The model under review builds one solid part; all positions refer to its coordinate system, in mm. Face numbers are marked on the shaded views. Give positions to 0.01 mm unless a question says otherwise; leave off trailing zeros. Order: outer loops, then holes, each group sorted by start corner. A loop starts at its lowest first (then second) coordinate and runs counter-clockwise, first axis right, second up.
Autodesk Inventor part; units mm, degrees
ref_plane "Work Plane1" through (-49.5, -19.63, -109) normal (0, 0, -1) x (0, 1, 0)
ref_plane "Work Plane2" through (-47.0185, 3.2145, -3.5) normal (1, 0, 0) x (0, 1, 0)
ref_plane "YZ Plane" through (0, 0, 0) normal (1, 0, 0) x (0, 1, 0)
sketch "Sketch1" plane through (0, 0, 0) normal (0, 0, 1) x (1, 0, 0)
  line L0 (47.5, 19.63) -> (-47.5, 19.63)
  arc A0 (-47.5, 19.63) -> (-49.5, 17.63) centre (-47.5, 17.63) ccw
  line L1 (-49.5, 17.63) -> (-49.5, -19.63)
  line L2 (49.5, -19.63) -> (49.5, 17.63)
  arc A1 (49.5, 17.63) -> (47.5, 19.63) centre (47.5, 17.63) ccw
  line L3 (-49.5, -19.63) -> (-52, -19.63)
  line L4 (-52, -19.63) -> (-52, 20.13)
  line L5 (-50, 22.13) -> (50, 22.13)
  line L6 (52, 20.13) -> (52, -19.63)
  line L7 (52, -19.63) -> (49.5, -19.63)
  arc A2 (-50, 22.13) -> (-52, 20.13) centre (-50, 20.13) ccw
  arc A3 (52, 20.13) -> (50, 22.13) centre (50, 20.13) ccw
  dimension "d0" = 2.5
  dimension "d1" = 2.5
  dimension "d2" = 2.5
  dimension "d3" = 2
ref_plane "Work Plane1" through (-49.5, -19.63, -109) normal (0, 0, -1) x (0, 1, 0)
extrude "Extrusion1" add sketch "Sketch1" against normal up to surface (109 mm away)
sketch "Sketch2" plane through (-50, 22.13, 0) normal (0, 1, 0) x (1, 0, 0)
  circle A0 centre (39.65, 50.5) radius 18.5 construction
  line L0 (58.85, 79.4) -> (20.45, 79.4) construction
  line L1 (20.45, 79.4) -> (20.45, 21.6) construction
  line L2 (58.85, 21.6) -> (58.85, 79.4) construction
  line L3 (20.45, 21.6) -> (58.85, 21.6) construction
  line L4 (20.15, 23.6) -> (20.15, 77.4) construction
  line L5 (59.15, 77.4) -> (59.15, 23.6) construction
  line L6 (20.15, 21.6) -> (59.15, 21.6) construction
  line L7 (59.15, 79.4) -> (20.15, 79.4) construction
  line L8 (20.15, 21.6) -> (59.15, 21.6)
  line L9 (59.15, 21.6) -> (59.15, 79.4)
  line L10 (59.15, 79.4) -> (20.15, 79.4)
  line L11 (20.15, 79.4) -> (20.15, 21.6)
  line L12 (59.65, 79.4) -> (19.65, 79.4)
  line L13 (19.65, 79.4) -> (19.65, 21.6)
  line L14 (19.65, 21.6) -> (59.65, 21.6)
  line L15 (59.65, 21.6) -> (59.65, 79.4)
  point P0 (50, 0)
  point P1 (59.65, 50.5)
  point P2 (59.15, 79.4)
  dimension "d43" = 40
  dimension "d44" = 39
  dimension "d45" = 0.5
extrude "Extrusion2" cut sketch "Sketch2" against normal up to surface (2.5 mm away)
chamfer "Chamfer1" distance 2.5 angle 45 4 edges at (-10.35, 22.13, -79.4) (-30.35, 22.13, -50.5) (9.65, 22.13, -50.5) (-10.35, 22.13, -21.6)
sketch "Sketch3" plane through (-52, -19.63, 0) normal (-1, 0, 0) x (0, 0, 1)
  line L0 (-94, 9.5) -> (-94, 37.26)
  arc A0 (-92, 39.26) -> (-94, 37.26) centre (-92, 37.26) ccw
  line L1 (-92, 39.26) -> (-17, 39.26)
  arc A1 (-15, 37.26) -> (-17, 39.26) centre (-17, 37.26) ccw
  line L2 (-15, 37.26) -> (-15, 9.5)
  line L3 (-94, 9.5) -> (-94, 0)
  line L4 (0, 0) -> (-109, 0) construction
  line L5 (-15, 9.5) -> (-15, 0)
  line L6 (-94, 0) -> (-15, 0)
  circle A2 centre (-98, 6.25) radius 1.5 construction
  circle A3 centre (-11, 6.25) radius 1.5 construction
  circle A4 centre (-98, 6.25) radius 1.75
  circle A5 centre (-11, 6.25) radius 1.75
  point P0 (0, 19.63)
  dimension "d13" = 3.5
  dimension "d14" = 3.5
ref_plane "Work Plane2" through (-47.0185, 3.2145, -3.5) normal (1, 0, 0) x (0, 1, 0)
extrude "Extrusion3" cut sketch "Sketch3" against normal up to surface (4.9815 mm away)
sketch "Sketch4" plane through (52, -19.63, 0) normal (1, 0, 0) x (0, 0, -1)
  circle A0 centre (98, 6.25) radius 1.5 construction
  circle A1 centre (11, 6.25) radius 1.5 construction
  arc A2 (72.9, 14.47) -> (72.9168, 14.38) centre (73.1508, 14.4702) ccw construction
  line L0 (72.9, 16.76) -> (72.9, 14.47) construction
  line L1 (72.9, 16.76) -> (72.9, 18.76) construction
  line L2 (72.9, 22.14) -> (72.9, 18.76) construction
  arc A3 (73.15, 22.39) -> (72.9, 22.14) centre (73.15, 22.14) ccw construction
  line L3 (73.15, 22.39) -> (85.55, 22.39) construction
  arc A4 (85.8, 22.14) -> (85.55, 22.39) centre (85.55, 22.14) ccw construction
  line L4 (85.8, 22.14) -> (85.8, 18.76) construction
  line L5 (85.8, 18.76) -> (85.8, 16.76) construction
  line L6 (85.8, 16.76) -> (85.8, 14.47) construction
  arc A5 (85.7832, 14.38) -> (85.8, 14.47) centre (85.5492, 14.4702) ccw construction
  line L7 (85.7832, 14.38) -> (86.5, 14.38) construction
  line L8 (86.5, 14.38) -> (86.5, 12.03) construction
  line L9 (81.88, 12.03) -> (86.5, 12.03) construction
  line L10 (81.88, 12.03) -> (81.88, 11.42) construction
  line L11 (81.88, 11.42) -> (86.45, 11.42) construction
  line L12 (87.2, 11.42) -> (86.45, 11.42) construction
  line L13 (87.2, 24.47) -> (87.2, 11.42) construction
  line L14 (87.2, 24.52) -> (87.2, 24.47) construction
  line L15 (87.2, 24.52) -> (71.7, 24.52) construction
  line L16 (71.7, 24.52) -> (71.7, 24.47) construction
  line L17 (71.7, 24.47) -> (71.7, 11.42) construction
  line L18 (71.7, 11.42) -> (72.45, 11.42) construction
  line L19 (72.45, 11.42) -> (76.82, 11.42) construction
  line L20 (76.82, 12.03) -> (76.82, 11.42) construction
  line L21 (72.3, 12.03) -> (76.82, 12.03) construction
  line L22 (72.3, 14.38) -> (72.3, 12.03) construction
  line L23 (72.3, 14.38) -> (72.9168, 14.38) construction
  line L24 (68.675, 20.9412) -> (68.975, 20.9412) construction
  line L25 (68.975, 20.9412) -> (68.975, 26.4362) construction
  arc A6 (68.975, 26.4362) -> (68.375, 27.0362) centre (68.375, 26.4362) ccw construction
  line L26 (68.375, 27.0362) -> (55.825, 27.0362) construction
  arc A7 (55.825, 27.0362) -> (55.225, 26.4362) centre (55.825, 26.4362) ccw construction
  line L27 (55.225, 26.4362) -> (55.225, 20.9412) construction
  line L28 (55.225, 20.9412) -> (55.525, 20.9412) construction
  line L29 (55.525, 26.4362) -> (55.525, 20.9412) construction
  arc A8 (55.825, 26.7362) -> (55.525, 26.4362) centre (55.825, 26.4362) ccw construction
  line L30 (68.375, 26.7362) -> (55.825, 26.7362) construction
  arc A9 (68.675, 26.4362) -> (68.375, 26.7362) centre (68.375, 26.4362) ccw construction
  line L31 (68.675, 26.4362) -> (68.675, 20.9412) construction
  line L32 (51.675, 20.9412) -> (51.975, 20.9412) construction
  line L33 (51.975, 20.9412) -> (51.975, 26.4362) construction
  arc A10 (51.975, 26.4362) -> (51.375, 27.0362) centre (51.375, 26.4362) ccw construction
  line L34 (51.375, 27.0362) -> (38.825, 27.0362) construction
  arc A11 (38.825, 27.0362) -> (38.225, 26.4362) centre (38.825, 26.4362) ccw construction
  line L35 (38.225, 26.4362) -> (38.225, 20.9412) construction
  line L36 (38.225, 20.9412) -> (38.525, 20.9412) construction
  line L37 (38.525, 26.4362) -> (38.525, 20.9412) construction
  arc A12 (38.825, 26.7362) -> (38.525, 26.4362) centre (38.825, 26.4362) ccw construction
  line L38 (51.375, 26.7362) -> (38.825, 26.7362) construction
  arc A13 (51.675, 26.4362) -> (51.375, 26.7362) centre (51.375, 26.4362) ccw construction
  line L39 (51.675, 26.4362) -> (51.675, 20.9412) construction
  line L40 (3.1, 11.07) -> (101.9, 11.07) construction
  circle A14 centre (8.5, 17.57) radius 4
  circle A15 centre (11, 6.25) radius 1.75
  circle A16 centre (98, 6.25) radius 1.75
  line L41 (37.975, 27.2862) -> (52.225, 27.2862)
  line L42 (52.225, 27.2862) -> (52.225, 10.82)
  line L43 (52.225, 10.82) -> (37.975, 10.82)
  line L44 (37.975, 10.82) -> (37.975, 27.2862)
  line L45 (54.975, 27.2862) -> (69.225, 27.2862)
  line L46 (69.225, 27.2862) -> (69.225, 10.82)
  line L47 (69.225, 10.82) -> (54.975, 10.82)
  line L48 (54.975, 10.82) -> (54.975, 27.2862)
  line L49 (71.45, 24.72) -> (87.45, 24.72)
  line L50 (87.45, 24.72) -> (87.45, 10.82)
  line L51 (87.45, 10.82) -> (71.45, 10.82)
  line L52 (71.45, 10.82) -> (71.45, 24.72)
  line L53 (90.5, 13.2962) -> (90.5, 12.7462) construction
  line L54 (91.35, 13.7962) -> (91, 13.7962) construction
  line L55 (98, 13.7962) -> (97.6, 13.7962) construction
  line L56 (98.5, 13.2962) -> (98.5, 12.7462) construction
  line L57 (89.75, 14.2962) -> (99.25, 14.2962)
  line L58 (99.25, 14.2962) -> (99.25, 10.57)
  line L59 (99.25, 10.57) -> (89.75, 10.57)
  line L60 (89.75, 10.57) -> (89.75, 14.2962)
  line L61 (71.7, 24.47) -> (87.2, 24.47) construction
  line L62 (87.2, 24.47) -> (87.2, 11.07) construction
  line L63 (87.2, 11.07) -> (71.7, 11.07) construction
  line L64 (71.7, 11.07) -> (71.7, 24.47) construction
  circle A17 centre (8.5, 17.57) radius 3.2
  line L65 (19.46, 17.8062) -> (32.46, 17.8062) construction
  line L66 (16.81, 16.0562) -> (16.81, 16.7062) construction
  line L67 (33.71, 16.5312) -> (33.71, 12.5212) construction
  line L68 (18.4564, 11.8926) -> (16.9564, 13.3926) construction
  line L69 (16.56, 17.8062) -> (33.96, 17.8062)
  line L70 (33.96, 17.8062) -> (33.96, 10.82)
  line L71 (33.96, 10.82) -> (19.1755, 10.82)
  line L72 (19.1755, 10.82) -> (16.56, 13.4355)
  line L73 (16.56, 13.4355) -> (16.56, 17.8062)
  point P0 (0, 19.63)
  point P1 (17.8, 27.1262)
  point P2 (68.975, 23.6887)
  point P3 (91.175, 13.7962)
  point P4 (90.5, 13.0212)
  point P5 (98.5, 13.0212)
  point P6 (16.81, 16.3812)
  dimension "d15" = 8
  dimension "d16" = 3.5
  dimension "d17" = 3.5
  dimension "d23" = 0.25
  dimension "d24" = 0.25
  dimension "d25" = 0.25
  dimension "d26" = 0.25
  dimension "d27" = 0.25
  dimension "d28" = 0.25
  dimension "d29" = 0.25
  dimension "d30" = 0.25
  dimension "d31" = 0.25
  dimension "d32" = 0.25
  dimension "d33" = 0.25
  dimension "d34" = 0.5
  dimension "d35" = 0.5
  dimension "d36" = 0.75
  dimension "d37" = 0.75
  dimension "d46" = 0.25
  dimension "d47" = 0.25
  dimension "d49" = 0.25
  dimension "d50" = 0.25
  dimension "d51" = 0.25
  dimension "d52" = 0
extrude "Extrusion4" cut sketch "Sketch4" against normal up to surface (2.5 mm away) contours A14 | A15 | A16 | L41 L42 L43 L44 | L45 L46 L47 L48 | L49 L50 L51 L52 | L57 L58 L59 L60 | A17 | L69 L70 L71 L72 L73
chamfer "Chamfer2" distance 2 angle 45 4 edges at (52, -13.38, -9.25) (52, -13.38, -96.25) (-52, -13.38, -99.75) (-52, -13.38, -12.75)
equation "\"d1\" = d0"
equation "\"d2\" = d0"
equation "\"d45\" = -0.5 * d44 + 0.5 * d43"
equation "\"d14\" = d13"
equation "\"d17\" = d16"
equation "\"d23\" = d20"
equation "\"d24\" = d23"
equation "\"d25\" = d24"
equation "\"d26\" = d24"
equation "\"d28\" = d26"
equation "\"d29\" = d25"
equation "\"d30\" = d29"
equation "\"d31\" = d27"
equation "\"d32\" = d31"
equation "\"d33\" = d31"
equation "\"d34\" = d35"
equation "\"d20\" = d18"
properties part number "Shroud Top"
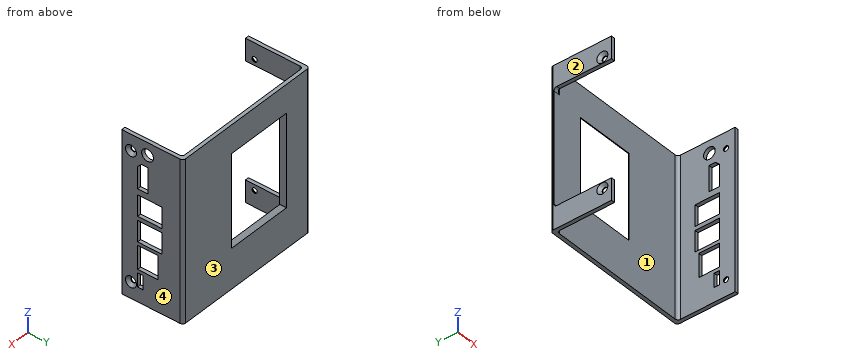
Item 1: Clearance check with flat-ended pins moving along their axes: pin 1 Ø1 at (x, z) = (28.5, -11.5) entering from -Y; pin 2 Ø5 at (y, z) = (-8.5, -75.5) entering from -X; pin 3 Ø0.8 at (x, z) = (50.5, -93) entering from +Y. State where each tip first meets the part, or that it passes through.
Values found:
pin 1: stops at y = 19.63
pin 2: stops at x = 49.5
pin 3: stops at y = 22.13
Item 2: Take a section at A-A (y = 15.5). Give the boundary of the cut face in (x, z).
Values found:
outline: (-52, -109) - (-49.5, -109) - (-49.5, -94) - (-52, -94) - close; (-52, -15) - (-49.5, -15) - (-49.5, 0) - (-52, 0) - close; (49.5, -109) - (52, -109) - (52, 0) - (49.5, 0) - close
Item 3: Take a section at B-B (z = -47). Give the number of separate pieces and of enclosed holes in the cut face, and give its area (3 significant figures).
Values found:
separate pieces: 3
enclosed holes: 0
area: 210 mm2
Item 4: Take a section at D-D (z = -11). Give the boundary of the cut face in (x, y).
Values found:
outline: (-52, -19.63) - (-49.5, -19.63) - (-49.5, -15.13) - (-50, -15.13) - (-52, -17.13) - close; (-52, -9.63) - (-50, -11.63) - (-49.5, -11.63) - (-49.5, 17.63) arc R2 cw to (-47.5, 19.63) - (47.5, 19.63) arc R2 cw to (49.5, 17.63) - (49.5, 1.06) - (52, 1.06) - (52, 20.13) arc R2 ccw to (50, 22.13) - (-50, 22.13) arc R2 ccw to (-52, 20.13) - close; (49.5, -19.63) - (52, -19.63) - (52, -17.13) - (50, -15.13) - (49.5, -15.13) - close; (49.5, -11.63) - (50, -11.63) - (52, -9.63) - (52, -5.18) - (49.5, -5.18) - close
Item 5: For line 1 (X direction, y = -17.5, z = -5.5); line 2 (X direction, y = -14.5, z = -18); line 3 (Y direction, x = 50, z = -8), list the stretches that pass through material, from the lowest coordinate up.
Values found:
line 1: x = -52 to -49.5, 49.5 to 52
line 2: x = 49.5 to 52
line 3: y = -19.63 to -6.03, 1.91 to 22.13
Item 6: Draft analysis for pull direction X (two halves, no side actions). For the marked faces 1, 2, 3 and 4, state which applies: released by +X, released by -X, zero draft, split by the parting line, or undercut.
Values found:
face 1: undercut
face 2: released by -X
face 3: zero draft
face 4: released by +X
